Check sheet for the drawn part. Datum: minimum x, y, z corner. Units: mm. A direction names the side the tool comes from. Coordinates: 2 decimals unless noted, no trailing zeros. Write each loop counter-clockwise with the first axis right and the second up, starting at its lowest first coordinate (ties: lowest second). Pieces come first, ordered by that corner, then holes. Notation, with made-up numbers: M -32,23.5 L -9,23.5 A32 cw -9,62.5 Z; hole C 17,-31 d2. An arc over 180 degrees is marked long. Write item = value, one per line. Start each with the question number.
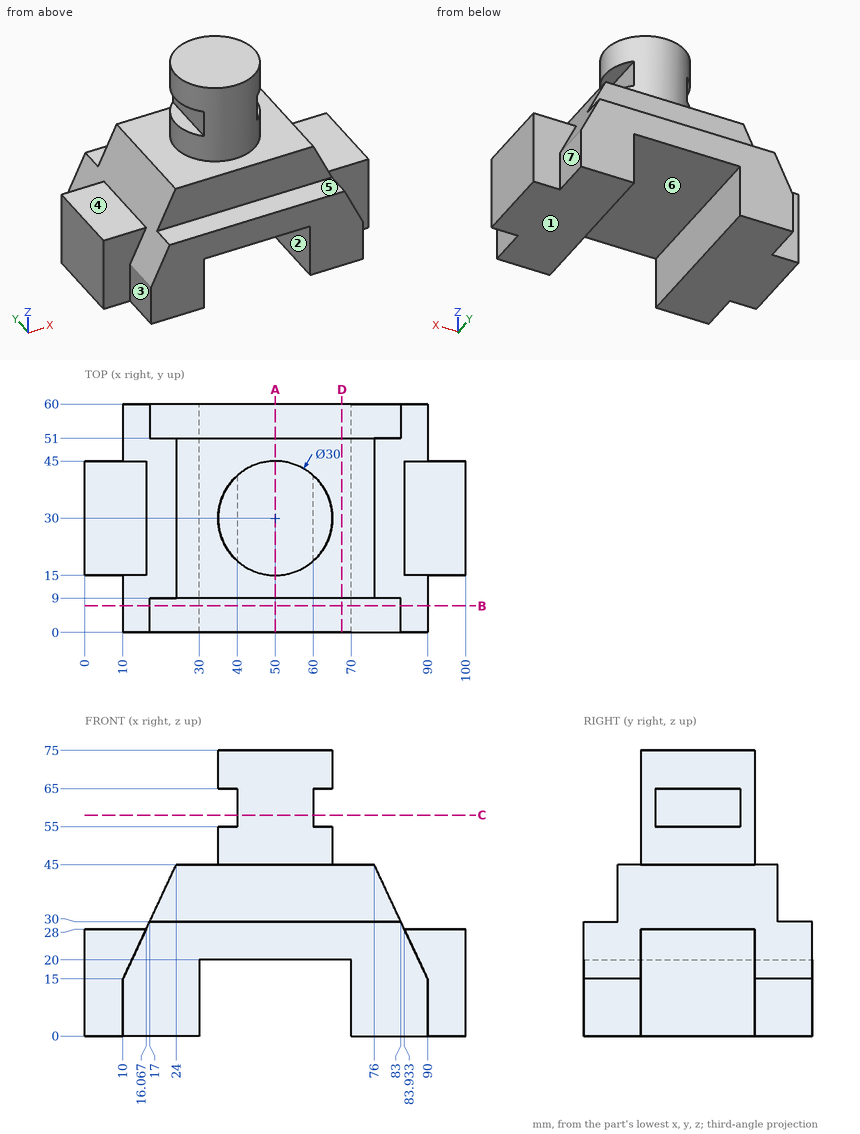
Q1. Draft check along X on the marked faces 1, 2 and 3. Enter one of: pulls with the +X half, pulls with the -X half, needs draft (parallel to the pull), parting line crosses it, or undercut.
Q2. Cross-section at B-B on y = 7. Enter the section's corners in (x, z), and give its area (4 significant figures).
Q3. Set-up check for the marked faces 4, 5, 6 and 7: record each of +Z, -Z, +X, -X, +Y, -Y from which the full face is reachable in a straight line by a thin tool's end or side.
Q4. Cross-section at D-D on x = 67.5. Enter the section's corners in (y, z), and give its area (3 significant figures).
Q5. Scan lines: L1, parallel to X at y = 32.5, z = 13.5; L2, parallel to Z at x = 35.5, y = 50; L3, parallel to Z at x = 16, y = 31. Record each from-to range of solid material in increasing order.
Q6. Cross-section at C-C on z = 58. Enter the section's corners in (x, y), and give its area (3 significant figures).
Q7. Gauge pin test, flat ends, axial feed: pin 1 (2 mm diameter, centred on x = 55, y = 8, fed in from -Z); pin 2 (5 mm diameter, centred on y = 49, z = 67, fed in from +X); pin 3 (16.5 mm diameter, centred on x = 39.5, z = 40.5, fed in from +Y); pin 4 (16.5 mm diameter, centred on y = 53, z = 5.5, fed in from +X). Record the tip position at first contact, or that the pin passes through.
Q8. Cross-section at A-A on x = 50. Enter the section's corners in (y, z), and give its area (3 significant figures).
Values found:
q1.face_1 = needs draft
q1.face_2 = undercut
q1.face_3 = pulls with the -X half
q2.outline = M 10,0 L 30,0 L 30,20 L 70,20 L 70,0 L 90,0 L 90,15 L 83,30 L 17,30 L 10,15 Z
q2.area = 1,495 mm²
q3.face_4 = +Z, -X, +Y, -Y
q3.face_5 = +Z, +X, -X, -Y
q3.face_6 = -Z, +Y, -Y
q3.face_7 = +Z, -Z, +X, +Y
q4.outline = M 0,20 L 60,20 L 60,30 L 51,30 L 51,45 L 9,45 L 9,30 L 0,30 Z
q4.area = 1,230 mm²
q5.L1 = 0 to 30, 70 to 100
q5.L2 = 20 to 45
q5.L3 = 0 to 28
q6.outline = M 40,18.82 A15 ccw 60,18.82 L 60,41.18 A15 ccw 40,41.18 Z
q6.area = 552 mm²
q7.pin_1 = 20
q7.pin_2 = through
q7.pin_3 = 51
q7.pin_4 = 100
q8.outline = M 0,20 L 60,20 L 60,30 L 51,30 L 51,45 L 45,45 L 45,75 L 15,75 L 15,45 L 9,45 L 9,30 L 0,30 Z
q8.area = 2,130 mm²
